Work out the finished part from the listing and answer in its coordinate system (mm). Round coordinates to 2 decimals unless told otherwise and drop trailing zeros. Order: outer loops, then holes, each group sorted by start corner. A loop starts at its lowest first (then second) coordinate and runs counter-clockwise, first axis right, second up. Notation, with made-up numbers: (-24.5, 55) - (28.5, 55) arc R11 ccw to (28.5, 76) - close; hole circle Ø9 at (-37, 41). An arc over 180 degrees is marked (long way). One line per question, with ' | ' between items. Start each with the question number.
from build123d import *

# Parameters (mm, degrees)
SKETCH1_W           = 255
SKETCH1_H           = 100
BOSS_EXTRUDE1_DEPTH = 1.5
SKETCH2_R           = 1.5
CUT_EXTRUDE2_DEPTH  = 10
SKETCH4_R           = 4
CUT_EXTRUDE3_DEPTH  = 137.961673471


with BuildPart() as part:
    # Sketch1 → Boss-Extrude1 (new body)
    with BuildSketch(Plane(origin=(0, 0, 0), x_dir=(1, 0, 0), z_dir=(0, 1, 0))):
        Rectangle(SKETCH1_W, SKETCH1_H)
    extrude(amount=BOSS_EXTRUDE1_DEPTH)

    # Sketch2 → Cut-Extrude2 (cut)
    with BuildSketch(Plane(origin=(0, 1.5, 0), x_dir=(1, 0, 0), z_dir=(0, 1, 0))):
        with Locations(Location((117.5, 40, 0), (0, 0, 270))):
            Circle(SKETCH2_R)
        with Locations(Location((97.5, 40, 0), (0, 0, 270))):
            Circle(SKETCH2_R)
        with Locations(Location((97.5, -40, 0), (0, 0, 270))):
            Circle(SKETCH2_R)
        with Locations(Location((117.5, -40, 0), (0, 0, 270))):
            Circle(SKETCH2_R)
        with Locations(Location((-97.5, 40, 0), (0, 0, 270))):
            Circle(SKETCH2_R)
        with Locations(Location((-117.5, 40, 0), (0, 0, 270))):
            Circle(SKETCH2_R)
        with Locations(Location((-117.5, -40, 0), (0, 0, 270))):
            Circle(SKETCH2_R)
        with Locations(Location((-97.5, -40, 0), (0, 0, 270))):
            Circle(SKETCH2_R)
    extrude(amount=-CUT_EXTRUDE2_DEPTH, mode=Mode.SUBTRACT)

    # Sketch4 → Cut-Extrude3 (cut, through all)
    with BuildSketch(Plane(origin=(0, 1.5, 0), x_dir=(1, 0, 0), z_dir=(0, 1, 0))):
        with Locations(Location((95.5, 15, 0), (0, 0, 270))):
            Circle(SKETCH4_R)
        with Locations(Location((-4.5, 35, 0), (0, 0, 270))):
            Circle(SKETCH4_R)
        with Locations(Location((-4.5, -5, 0), (0, 0, 270))):
            Circle(SKETCH4_R)
    extrude(amount=-CUT_EXTRUDE3_DEPTH, mode=Mode.SUBTRACT)


solid = part.part
1) Straight lines are drawn through the part: line 1 (Z direction, x = -117.5, y = 1); line 2 (X direction, y = 0.55, z = 40); line 3 (X direction, y = 1.2, z = 4.5). For each, find the intervals that lie inside material, in ascending order.
2) Determine the mould class of faces 1 (the cylindrical face through (91.595, 0.76, -15.867)), 2 (the flat face through (-2, 0, -1)) for opening direction X: released by +X, released by -X, zero draft, split by the parting line, or undercut.
3) Section A-A on z = 5 is taken. Give the vertices of the cut face in (x, y).
4) Section B-B on x = -4.5 is taken. Give the vertices of the cut face in (y, z).
5) A flat-ended cylindrical pin translates along its axis: pin 1 (3.5 mm diameter, centred on x = 97.5, z = 40, fed in from -Y). Find the tip coordinate at first contact, or state that the pin passes through.
Recorded:
1) line 1: z = -50 to -41.5, -38.5 to 38.5, 41.5 to 50 | line 2: x = -127.5 to -119, -116 to -99, -96 to 96, 99 to 116, 119 to 127.5 | line 3: x = -127.5 to -8.47, -0.53 to 127.5
2) face 1: undercut | face 2: zero draft
3) outline: (-127.5, 0) - (-8.5, 0) - (-8.5, 1.5) - (-127.5, 1.5) - close; (-0.5, 0) - (127.5, 0) - (127.5, 1.5) - (-0.5, 1.5) - close
4) outline: (0, -50) - (1.5, -50) - (1.5, -39) - (0, -39) - close; (0, -31) - (1.5, -31) - (1.5, 1) - (0, 1) - close; (0, 9) - (1.5, 9) - (1.5, 50) - (0, 50) - close
5) pin 1: stops at y = 0
